from build123d import *

# Parameters (mm, degrees)
F1_DEPTH = 25.4
F2_R     = 12.7
F3_DEPTH = 25.4
F6_W     = 25.4
F6_H     = 254
F7_DEPTH = 25.4
F9_DEPTH = 12.7


with BuildPart() as f1:
    # F0 (on Top) → F1 (new body)
    with BuildSketch(Plane.XY):
        Polygon((-88.9, 0), (-63.5, 0), (-63.5, 76.2), (0, 76.2), (63.5, 76.2), (63.5, 0), (88.9, 0), (88.9, 101.6), (0, 101.6), (-88.9, 101.6), align=None)
    extrude(amount=F1_DEPTH)

    # F2 (on face) → F3 (join)
    with BuildSketch(Plane.YZ.offset(-63.5)):
        with Locations((12.6999979839, 12.7)):
            Circle(F2_R)
    extrude(amount=F3_DEPTH)

    # F4: F1 across plane


with BuildPart() as f1_1:
    add(f1.part)
    add(f1.part.mirror(Plane.YZ))

    # F6 (on face) → F7 (join)
    with BuildSketch(Plane(origin=(0, 25.4, -25.4), x_dir=(-1, 0, 0), z_dir=(0, 0.7071067812, -0.7071067812))):
        with Locations((38.1, 198.8420489686)):
            Rectangle(F6_W, F6_H)
    extrude(amount=F7_DEPTH)

    # F8 (on face) → F9 (join)
    with BuildSketch(Plane.YZ.offset(-25.4)):
        with BuildLine():
            ThreePointArc((264.7853785425, 178.0643540582), (267.5383924843, 182.1845305882), (268.5051224214, 187.0446101792))
            ThreePointArc((268.5051224214, 187.0446101792), (267.5383924843, 191.9046897703), (264.7853785425, 196.0248663003))
            ThreePointArc((264.7853785425, 196.0248663003), (255.8051224214, 199.7446101792), (246.8248663003, 196.0248663003))
            ThreePointArc((246.8248663003, 196.0248663003), (246.8248663003, 178.0643540582), (264.7853785425, 178.0643540582))
        make_face()
    extrude(amount=F9_DEPTH)

    # F10: F1 across plane


with BuildPart() as f1_2:
    add(f1_1.part)
    add(f1_1.part.mirror(Plane.YZ))


solid = f1_2.part
The model under review builds one solid part; all positions refer to its coordinate system, in mm. A direction names the side the tool comes from. Round coordinates to 2 decimals unless told otherwise and drop trailing zeros. Order: outer loops, then holes, each group sorted by start corner. A loop starts at its lowest first (then second) coordinate and runs counter-clockwise, first axis right, second up. Notation, with made-up numbers: (4, 77) -> (13, 77) arc R15 ccw to (13, 91) -> close; hole circle Ø1 at (69, -3.75). An arc over 180 degrees is marked (long way). Return JSON: item names as keys, results as strings.
1. For L1, parallel to X at y = 184, z = 108.5; L2, parallel to Z at x = 8, y = 89; L3, parallel to Z at x = -28.5, y = 173, list the stretches that pass through material, from the lowest coordinate up. Write a range as [from, to].
Answer block:
{"L1": "x = [-50.8, -25.4], [25.4, 50.8]", "L2": "z = [0, 25.4]", "L3": "z = [86.28, 122.2]"}
2. Insertion check: P1, Ø5, axis at y = 203, z = 119.5, coming from the -X side; P2, Ø10, axis at x = -23.5, y = 169.5, coming from the +Z side; P3, Ø12.5, axis at x = -29, z = 10, coming from the +Y side. Each pin has a flat end and moves straight along its axis. Give the tip position at first contact, or say it passes through.
Answer block:
{"P1": "stops at x = -50.8", "P2": "stops at z = 123.32", "P3": "stops at y = 102.97"}
3. The part is to be moulded in two halves that separate along Y. For faces 5 (the face through (1, 101.6, 13)), 6 (the face through (37.9, 167.3, 116.5)), 7 (the face through (-1, 76.2, 13)), 8 (the face through (38.1, 13, 13)), say which applies: +Y half, -Y half, draft (parallel to the pull), parting line (faces both ways), or undercut.
Answer block:
{"face 5": "+Y half", "face 6": "-Y half", "face 7": "undercut", "face 8": "draft"}
4. Take a section at B-B (y = 39). Write out the cut boundary in (x, z), then the cut area to 3 significant figures.
Answer block:
{"outline": "(-88.9, 0) -> (-63.5, 0) -> (-63.5, 25.4) -> (-88.9, 25.4) -> close; (63.5, 0) -> (88.9, 0) -> (88.9, 25.4) -> (63.5, 25.4) -> close", "area": "1,290 mm²"}
5. Take a section at C-C (z = 77). Write out the cut boundary in (x, y), then the cut area to 3 significant figures.
Answer block:
{"outline": "(-50.8, 127.8) -> (-25.4, 127.8) -> (-25.4, 163.72) -> (-50.8, 163.72) -> close; (25.4, 127.8) -> (50.8, 127.8) -> (50.8, 163.72) -> (25.4, 163.72) -> close", "area": "1,820 mm²"}
6. Take a section at D-D (x = 1). Write out the cut boundary in (y, z).
Answer block:
{"outline": "(76.2, 0) -> (101.6, 0) -> (101.6, 25.4) -> (76.2, 25.4) -> close"}
7. Take a section at A-A (x = -44.5). Write out the cut boundary in (y, z), then the cut area to 3 significant figures.
Answer block:
{"outline": "circle Ø25.4 at (12.7, 12.7); (76.2, 0) -> (101.6, 0) -> (101.6, 14.88) -> (273.77, 187.04) -> (255.81, 205.01) -> (76.2, 25.4) -> close", "area": "7,340 mm²"}
8. For faces 1 (the face through (-50.978, 19.527, 23.409)), 2 (the face through (-63.5, 3, 22)), 3 (the face through (-63.5, 3, 3)), 4 (the face through (-74, 52, 25.4)), list the 3-axis set-ups (+Z, -Z, +X, -X, +Y, -Y) from which the entire face can be reached by the end or side of a thin tool; tool diameter is ignored.
Answer block:
{"face 1": "none", "face 2": "+Z, -Y", "face 3": "-Z, -Y", "face 4": "+Z, -X, +Y, -Y"}
